Input: part model. Units: mm. Frame: model coordinates. Face numbers are marked on the shaded views. A direction names the side the tool comes from. Coordinates: 2 decimals unless noted, no trailing zeros. Order: outer loops, then holes, each group sorted by start corner. A loop starts at its lowest first (then second) coordinate and runs counter-clockwise, first axis right, second up. Notation, with made-up numbers: (0, 68) - (45, 68) arc R36 ccw to (45, 105) - close; hole circle Ø2 at (64.5, 14.5). An arc over 180 degrees is marked (long way). One line per question, with ' | ' between items. Start each with the question number.
```python
from build123d import *

# Parameters (mm, degrees)
F0_W     = 12.7
F0_H     = 4.7625
F2_DEPTH = 1.5875
F3_R     = 6.35


with BuildPart() as f1:
    # F0 (on Top) → F1 (revolve)
    with BuildSketch(Plane.XY):
        with Locations((-50.996662, 30.11827)):
            Rectangle(F0_W, F0_H)
        Polygon((37.903338, 32.49952), (-44.646662, 32.49952), (-44.646662, 27.73702), (47.555338, 27.73702), (47.555338, 29.32452), (37.903338, 29.32452), align=None)
    revolve(axis=Axis((1.454338, 27.73702, 0), (-1, 0, 0)))

    # F0 (on Top) → F2 (join, symmetric)
    with BuildSketch(Plane.XY):
        Polygon((-44.646662, 22.97452), (-44.646662, 27.73702), (-57.346662, 27.73702), (-57.346662, 11.86202), (-44.646662, 11.86202), align=None)
    extrude(amount=F2_DEPTH, both=True)

    # F3
    f3_edges = [f1.edges().sort_by_distance(p)[0] for p in [
        (-57.346662, 11.86202, 0),
    ]]
    fillet(f3_edges, radius=F3_R)


solid = f1.part
```
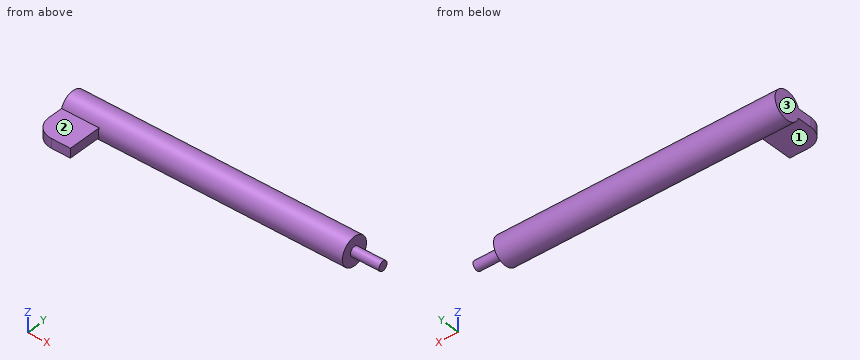
(1) Material intervals for line 1 along X through (y, z) = (25, 2.5); line 2 along Y through (x, z) = (12, -0.25); line 3 along Y through (x, z) = (27, -0.75), sorted ascending. Write a range as from..to.
(2) Reachability of the marked faces 1, 2 and 3 from +Z, -Z, +X, -X, +Y, -Y: full face, straight path, thin tool, end or side. Return the list, or none.
(3) Pin query (flat end, axial travel): pin 1 (8 mm diameter, centred on x = 28, y = 17.5, fed in from +Z); pin 2 (6 mm diameter, centred on x = 17, y = 22, fed in from -Z); pin 3 (1 mm diameter, centred on y = 25, z = 1, fed in from +X); pin 4 (1.6 mm diameter, centred on y = 19.5, z = 1, fed in from +X). Return the tip coordinate at first contact, or that it passes through.
(4) Section A-A (z = 0). Output: boundary loops of the cut face in (x, y).
(5) Section D-D (y = 30.25). Output: boundary loops of the cut face in (x, z).
(6) Section B-B (y = 19.5). Output: boundary loops of the cut face in (x, z), then the cut area to 3 significant figures.
(7) Section C-C (x = 27). Output: boundary loops of the cut face in (y, z) (1 decimal).
Worked answers:
1) line 1: x = -57.35..37.9 | line 2: y = 22.98..32.49 | line 3: y = 23.03..32.44
2) face 1: -Z, +X, -X, -Y | face 2: +Z, +X, -X, -Y | face 3: +Z, -Z, -X, +Y, -Y
3) pin 1: passes through | pin 2: stops at z = -3.9 | pin 3: stops at x = 37.9 | pin 4: stops at x = -44.65
4) outline: (-57.35, 18.21) arc R6.35 ccw to (-51, 11.86) - (-44.65, 11.86) - (-44.65, 22.97) - (37.9, 22.97) - (37.9, 26.15) - (47.56, 26.15) - (47.56, 29.32) - (37.9, 29.32) - (37.9, 32.5) - (-57.35, 32.5) - close
5) outline: (-57.35, -4.05) - (37.9, -4.05) - (37.9, 4.05) - (-57.35, 4.05) - close
6) outline: (-57.35, -1.59) - (-44.65, -1.59) - (-44.65, 1.59) - (-57.35, 1.59) - close | area: 40.3 mm²
7) outline: circle Ø9.5 at (27.7, 0)
